Part model, mm, in its own coordinate system. A direction names the side the tool comes from. Coordinates: 2 decimals unless noted, no trailing zeros. Loops run counter-clockwise (first coordinate to the right, second up) from the corner with the lowest first, then second, coordinate; pieces in that order, holes last. Notation, with made-up numbers: M 84.25,-28 L 129.25,-28 A28 ccw 129.25,-7 Z; hole C -37,31 d7. An arc over 180 degrees is marked long. Answer as a JSON object with one key per item and string values. Group by question number.
1. Drop flat-ended pins along their axis: pin 1 Ø1 at (x, z) = (2, -1.5) entering from -Y; pin 2 Ø1.8 at (x, z) = (0, 0) entering from +Y; pin 3 Ø1.5 at (x, y) = (-2, 4.5) entering from +Z. Give the stop position or say it passes through.
2. Saw through at C-C on y = 3.5. Write the cut outline in (x, z).
3. Mould opens along Z. For faces 1 (the face through (-0.45, 4.78, -1.43)), 2 (the face through (0, -4.5, 0)), 3 (the face through (0, 2.5, 0)), 4 (the face through (0.45, -2.22, -1.43)) say: released by +Z, released by -Z, zero draft, split by the parting line, or undercut.
4. Drill centre lines: L1, parallel to X at y = 5.15, z = 0; L2, parallel to Y at x = -2.1, z = 1.65; L3, parallel to X at y = 4.75, z = 1. Where is each one in solid material? Low to high.
5. Saw through at D-D on y = 2.25. Write the cut outline in (x, z).
6. Saw through at B-B on x = 0. Write the cut outline in (y, z), then the cut area to 3 significant figures.
7. Saw through at A-A on z = 0. Write the cut outline in (x, y), then the cut area to 3 significant figures.
8. 3-axis set-ups, long thin cutter, end or side, ignore diameter. For faces 5 (the face through (-1.2, 0, 1.2)), 6 (the face through (-1.2, 7, 1.2)): which of +Z, -Z, +X, -X, +Y, -Y reach the whole face in a straight line?
from build123d import *

# Parameters (mm, degrees)
SKETCH1_R           = 2.9
BOSS_EXTRUDE1_DEPTH = 7
SKETCH2_R           = 1.5
BOSS_EXTRUDE2_DEPTH = 4.5
SKETCH3_R           = 1.5
CUT_EXTRUDE1_DEPTH  = 4.5


with BuildPart() as part:
    # Sketch1 → Boss-Extrude1 (new body)
    with BuildSketch(Plane(origin=(0, 0, 0), x_dir=(1, 0, 0), z_dir=(0, 1, 0))):
        with Locations(Location((0, 0, 0), (0, 0, 270))):
            Circle(SKETCH1_R)
    extrude(amount=BOSS_EXTRUDE1_DEPTH)

    # Sketch2 → Boss-Extrude2 (add)
    with BuildSketch(Plane.XZ):
        with Locations(Location((0, 0, 0), (0, 0, 270))):
            Circle(SKETCH2_R)
    extrude(amount=BOSS_EXTRUDE2_DEPTH)

    # Sketch3 → Cut-Extrude1 (cut)
    with BuildSketch(Plane(origin=(0, 7, 0), x_dir=(1, 0, 0), z_dir=(0, 1, 0))):
        with Locations(Location((0, 0, 0), (0, 0, 90))):
            Circle(SKETCH3_R)
    extrude(amount=-CUT_EXTRUDE1_DEPTH, mode=Mode.SUBTRACT)


solid = part.part
Outcome:
{
 "1": {"pin 1": "stops at y = 0", "pin 2": "stops at y = 2.5", "pin 3": "stops at z = 2.62"},
 "2": {"outline": "C 0,0 d5.8; hole C 0,0 d3"},
 "3": {"face 1": "undercut", "face 2": "zero draft", "face 3": "undercut", "face 4": "split by the parting line"},
 "4": {"L1": "x = -2.9 to -1.5, 1.5 to 2.9", "L2": "y = 0 to 7", "L3": "x = -2.72 to -1.12, 1.12 to 2.72"},
 "5": {"outline": "C 0,0 d5.8"},
 "6": {"outline": "M -4.5,-1.5 L 0,-1.5 L 0,-2.9 L 7,-2.9 L 7,-1.5 L 2.5,-1.5 L 2.5,1.5 L 7,1.5 L 7,2.9 L 0,2.9 L 0,1.5 L -4.5,1.5 Z", "area": "40.6 mm²"},
 "7": {"outline": "M -2.9,0 L -1.5,0 L -1.5,-4.5 L 1.5,-4.5 L 1.5,0 L 2.9,0 L 2.9,7 L 1.5,7 L 1.5,2.5 L -1.5,2.5 L -1.5,7 L -2.9,7 Z", "area": "40.6 mm²"},
 "8": {"face 5": "-Y", "face 6": "+Z, -Z, +X, -X, +Y"}
}
